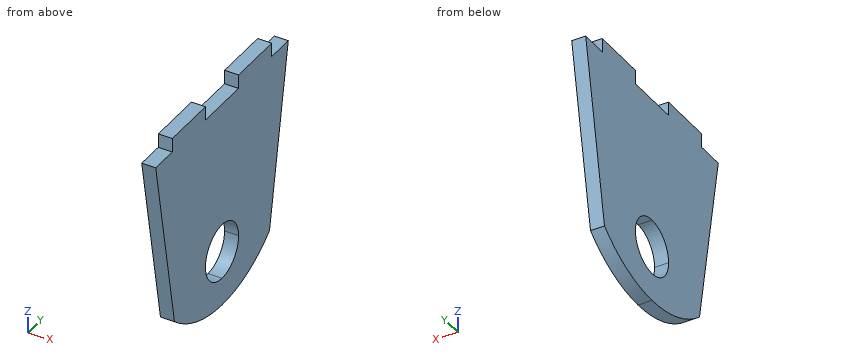
```python
from build123d import *

# Parameters (mm, degrees)
F1_DEPTH = 6.35
F2_W     = 12.7
F2_H     = 6.35
F3_DEPTH = 25.4
F5_DEPTH = 6.351


# Not quite as in the source:
# - a feature names something its author has since deleted; it is built from what else it names


with BuildPart() as f1:
    # F0 (on Right) → F1 (new body)
    with BuildSketch(Plane.YZ):
        with BuildLine():
            Line((50.8, 0), (0, 0))
            Line((0, 0), (0, -6.35))
            Line((0, -6.35), (14.3783799252, -87.8938446653))
            ThreePointArc((14.3783799252, -87.8938446653), (31.3423979963, -98.0600456848), (50.8, -101.6))
            Line((50.8, -101.6), (50.8, 0))
        make_face()
        with BuildLine():
            Line((101.6, 0), (50.8, 0))
            Line((50.8, 0), (50.8, -101.6))
            ThreePointArc((50.8, -101.6), (70.2576020037, -98.0600456848), (87.2216200748, -87.8938446653))
            Line((87.2216200748, -87.8938446653), (101.6, -6.35))
            Line((101.6, -6.35), (101.6, 0))
        make_face()
    extrude(amount=F1_DEPTH)

    # F2 (on face) → F3 (cut)
    with BuildSketch(Plane.YZ.offset(6.35)):
        with Locations((95.25, -3.175)):
            Rectangle(F2_W, F2_H)
        with Locations((44.45, -3.175)):
            Rectangle(F2_W, F2_H)
        with Locations((6.35, -3.175)):
            Rectangle(F2_W, F2_H)
        with Locations((57.15, -3.175)):
            Rectangle(F2_W, F2_H)
    extrude(amount=-F3_DEPTH, mode=Mode.SUBTRACT)

    # F4 (on face) → F5 (cut, through all)
    with BuildSketch(Plane.YZ.offset(6.35)):
        with BuildLine():
            Line((50.8, -88.9), (50.8, -76.2))
            Line((50.8, -76.2), (38.1, -76.2))
            ThreePointArc((38.1, -76.2), (41.8197438789, -85.1802561211), (50.8, -88.9))
        make_face()
        with BuildLine():
            Line((50.8, -76.2), (63.5, -76.2))
            ThreePointArc((63.5, -76.2), (59.7802561211, -67.2197438789), (50.8, -63.5))
            Line((50.8, -63.5), (50.8, -76.2))
        make_face()
        with BuildLine():
            ThreePointArc((50.8, -88.9), (59.7802561211, -85.1802561211), (63.5, -76.2))
            Line((63.5, -76.2), (50.8, -76.2))
            Line((50.8, -76.2), (50.8, -88.9))
        make_face()
        with BuildLine():
            Line((38.1, -76.2), (50.8, -76.2))
            Line((50.8, -76.2), (50.8, -63.5))
            ThreePointArc((50.8, -63.5), (41.8197438789, -67.2197438789), (38.1, -76.2))
        make_face()
    extrude(amount=-F5_DEPTH, mode=Mode.SUBTRACT)


solid = f1.part
```
The model under review builds one solid part; all positions refer to its coordinate system, in mm. Round coordinates to 2 decimals unless told otherwise and drop trailing zeros. Order: outer loops, then holes, each group sorted by start corner. A loop starts at its lowest first (then second) coordinate and runs counter-clockwise, first axis right, second up. Notation, with made-up numbers: M -6,-31 L 13,-31 A28 cw 13,-12 Z; hole C 62.5,38.25 d9. An arc over 180 degrees is marked long. Use a Markdown table: item, result.
1) Consider section A-A (x = 3). Write out the cut boundary in (y, z) (3 decimals).
Report:
| item | result |
|---|---|
| outline | M 0,-6.35 L 14.378,-87.894 A55.245 ccw 87.222,-87.894 L 101.6,-6.35 L 88.9,-6.35 L 88.9,0 L 63.5,0 L 63.5,-6.35 L 38.1,-6.35 L 38.1,0 L 12.7,0 L 12.7,-6.35 Z; hole C 50.8,-76.2 d25.4 |
2) Consider section B-B (y = 59.5). Write out the cut boundary in (x, z).
Report:
| item | result |
|---|---|
| outline | M 0,-100.91 L 6.35,-100.91 L 6.35,-85.45 L 0,-85.45 Z; M 0,-66.95 L 6.35,-66.95 L 6.35,-6.35 L 0,-6.35 Z |
3) Wall thickness on line 1 along Y through (x, z) = (2, -6); line 2 along Y through (x, z) = (1.5, -76); line 3 along Z through (x, y) = (4, 47.5): over which ranges is each line inside the solid? List them lowest first. Write a range as [from, to].
Report:
| item | result |
|---|---|
| line 1 | [12.7, 38.1], [63.5, 88.9] |
| line 2 | [12.28, 38.1], [63.5, 89.32] |
| line 3 | [-101.5, -88.46], [-63.94, -6.35] |
4) Consider section D-D (y = 73.5). Write out the cut boundary in (x, z), then the cut area to 3 significant figures.
Report:
| item | result |
|---|---|
| outline | M 0,-96.72 L 6.35,-96.72 L 6.35,0 L 0,0 Z |
| area | 614 mm^2 |
5) Consider section C-C (z = -71.5). Write out the cut boundary in (x, y).
Report:
| item | result |
|---|---|
| outline | M 0,11.49 L 6.35,11.49 L 6.35,39 L 0,39 Z; M 0,62.6 L 6.35,62.6 L 6.35,90.11 L 0,90.11 Z |
6) Insertion check: pin 1 (1 mm diameter, centred on x = 4, z = -16.5, fed in from -Y); pin 2 (1.9 mm diameter, centred on x = 4, z = -1.5, fed in from -Y). Each pin has a flat end and moves straight along its axis. Give the tip position at first contact, or say it passes through.
Report:
| item | result |
|---|---|
| pin 1 | y = 1.7 |
| pin 2 | y = 12.7 |
